```python
from build123d import *

# Parameters (mm, degrees)
SKETCH1_W           = 26.67
SKETCH1_H           = 12.7
BOARD_OUTLINE_DEPTH = 1.6
SKETCH2_R           = 0.254
NPTH_DEPTH          = 30.582746661
SKETCH3_R           = 0.51
PTH_DEPTH           = 30.582746661


with BuildPart() as part:
    # Sketch1 → Board_Outline (new body)
    with BuildSketch(Plane.XY):
        with Locations((13.335, 6.35)):
            Rectangle(SKETCH1_W, SKETCH1_H)
    extrude(amount=BOARD_OUTLINE_DEPTH)

    # Sketch2 → NPTH (cut, through all)
    with BuildSketch(Plane.XY):
        with Locations((8.7122, 7.5946)):
            Circle(SKETCH2_R)
        with Locations((10.0076, 7.62)):
            Circle(SKETCH2_R)
        with Locations((13.3096, 9.8298)):
            Circle(SKETCH2_R)
        with Locations((20.9042, 11.43)):
            Circle(SKETCH2_R)
        with Locations((4.8768, 8.9662)):
            Circle(SKETCH2_R)
    extrude(amount=NPTH_DEPTH, mode=Mode.SUBTRACT)

    # Sketch3 → PTH (cut, through all)
    with BuildSketch(Plane.XY):
        with Locations((1.27, 7.62)):
            Circle(SKETCH3_R)
        with Locations((1.27, 5.08)):
            Circle(SKETCH3_R)
        with Locations((15.24, 7.62)):
            Circle(SKETCH3_R)
        with Locations((15.24, 5.08)):
            Circle(SKETCH3_R)
    extrude(amount=PTH_DEPTH, mode=Mode.SUBTRACT)


solid = part.part
```
Verification items for the finished model (mm, model axes). Coordinates: 2 decimals unless noted, no trailing zeros. Loops run counter-clockwise (first coordinate to the right, second up) from the corner with the lowest first, then second, coordinate; pieces in that order, holes last. Notation, with made-up numbers: (60, -36) -> (108, -36) arc R15 cw to (108, -11) -> close; hole circle Ø4 at (13, 44). An arc over 180 degrees is marked (long way). Answer in a Markdown table with one row per item. Add a question column.
1. Draft check along X on faces 1 (the face through (15.514, 5.51, 0.789)), 2 (the face through (13, 12.7, 1)), 3 (the face through (0, 6, 1)). Enter one of: +X half, -X half, draft (parallel to the pull), parting line (faces both ways), or undercut.
2. Section check A-A, the plane x = 1.27. Enter the section's corners in (y, z), then the cut area to 3 significant figures.
3. Material ranges on probe 1 along X at (y, z) = (5.08, 0.55); probe 2 along X at (y, z) = (7.62, 1.35); probe 3 along Y at (x, z) = (1.27, 0.8), recorded low to high. Write a range as [from, to].
4. Depth check by flat-ended pin: P1, Ø3, axis at x = 18.5, y = 8.5, coming from the -Z side. Enter the tip coordinate at first touch or a pass-through.
Derived:
| question | item | result |
|---|---|---|
| 1 | face 1 | undercut |
| 1 | face 2 | draft |
| 1 | face 3 | -X half |
| 2 | outline | (0, 0) -> (4.57, 0) -> (4.57, 1.6) -> (0, 1.6) -> close; (5.59, 0) -> (7.11, 0) -> (7.11, 1.6) -> (5.59, 1.6) -> close; (8.13, 0) -> (12.7, 0) -> (12.7, 1.6) -> (8.13, 1.6) -> close |
| 2 | area | 17.1 mm² |
| 3 | probe 1 | x = [0, 0.76], [1.78, 14.73], [15.75, 26.67] |
| 3 | probe 2 | x = [0, 0.76], [1.78, 8.46], [8.96, 9.75], [10.26, 14.73], [15.75, 26.67] |
| 3 | probe 3 | y = [0, 4.57], [5.59, 7.11], [8.13, 12.7] |
| 4 | P1 | stops at z = 0 |
